Could you check a few things on this model? Use its own coordinates, in mm. A direction names the side the tool comes from. Round coordinates to 2 decimals unless told otherwise and drop trailing zeros. Loops run counter-clockwise (first coordinate to the right, second up) from the corner with the lowest first, then second, coordinate; pieces in that order, holes last.
from build123d import *

# Parameters (mm, degrees)
BOX_W           = 200
BOX_H           = 200
BOX_DEPTH       = 200
SKETCH_W        = 170.31563
SKETCH_H        = 140.120693
SKETCH_W_2      = 170.274007
SKETCH_H_2      = 27.404772
POCKET_DEPTH    = 180
SKETCH001_R     = 6
POCKET004_DEPTH = 20


with BuildPart() as part:
    # Box → Box (new body)
    with BuildSketch(Plane.XY):
        with Locations((100, 100)):
            Rectangle(BOX_W, BOX_H)
    extrude(amount=BOX_DEPTH)

    # Sketch → Pocket (cut)
    with BuildSketch(Plane.XZ):
        with Locations((99.987303, 117.884569)):
            Rectangle(SKETCH_W, SKETCH_H)
        with Locations((99.992803, 27.16207)):
            Rectangle(SKETCH_W_2, SKETCH_H_2)
    extrude(amount=-POCKET_DEPTH, mode=Mode.SUBTRACT)

    # Sketch001 → Pocket004 (cut)
    with BuildSketch(Plane.YZ.offset(200)):
        with Locations((130.008312, 66.836238)):
            Circle(SKETCH001_R)
        with Locations((160.008312, 66.836238)):
            Circle(SKETCH001_R)
    extrude(amount=-POCKET004_DEPTH, mode=Mode.SUBTRACT)


solid = part.part
Item 1: For faces 5 (the flat face through (99, 89, 187.945)), 6 (the flat face through (99, 101, 0)), 7 (the cylindrical face through (192.677, 155.247, 63.185)), which set-ups out of +Z, -Z, +X, -X, +Y, -Y let a thin tool reach every point of the face, with its end or its side?
Results list:
face 5: -Y
face 6: -Z, +X, -X, +Y, -Y
face 7: +X
Item 2: If we section it at A-A, the plane y = 133: Please give me the cut outline in (x, z).
Results list:
outline: (0, 0) - (200, 0) - (200, 61.64) - (185.15, 61.64) - (185.15, 47.82) - (14.83, 47.82) - (14.83, 187.94) - (185.15, 187.94) - (185.15, 72.04) - (200, 72.04) - (200, 200) - (0, 200) - close; hole (14.86, 13.46) - (185.13, 13.46) - (185.13, 40.86) - (14.86, 40.86) - close
Item 3: If I drill on line 1 along Z through (x, y) = (71, 68); line 2 along X through (y, z) = (81.5, 105); line 3 along X through (y, z) = (161, 17), over which ranges is the centre line in solid material (lowest first)?
Results list:
line 1: z = 0 to 13.46, 40.86 to 47.82, 187.94 to 200
line 2: x = 0 to 14.83, 185.15 to 200
line 3: x = 0 to 14.86, 185.13 to 200
Item 4: Will this pin go through, and if not, where does the flat tip stop? pin 1 (12 mm diameter, centred on x = 171.5, z = 149, fed in from -Y).
Results list:
pin 1: stops at y = 180
Item 5: If we section it at D-D, the plane z = 16.5: Please give me the cut outline in (x, y).
Results list:
outline: (0, 0) - (14.86, 0) - (14.86, 180) - (185.13, 180) - (185.13, 0) - (200, 0) - (200, 200) - (0, 200) - close
Item 6: If we section it at C-C, the plane z = 139: Please give me the cut outline in (x, y), then the cut area to 3 significant figures.
Results list:
outline: (0, 0) - (14.83, 0) - (14.83, 180) - (185.15, 180) - (185.15, 0) - (200, 0) - (200, 200) - (0, 200) - close
area: 9,340 mm2
Item 7: We'd pull the mould along Z, two halves only. Please class faces 1 (the flat face through (0, 99, 99)), 2 (the flat face through (99, 101, 200)), 3 (the cylindrical face through (192.677, 124.014, 67.1)), 4 (the flat face through (14.856, 89, 27)): released by +Z, released by -Z, zero draft, split by the parting line, or undercut.
Results list:
face 1: zero draft
face 2: released by +Z
face 3: undercut
face 4: undercut
Item 8: If we section it at B-B, the plane x = 21: Please give me the cut outline in (y, z).
Results list:
outline: (0, 0) - (200, 0) - (200, 200) - (0, 200) - (0, 187.94) - (180, 187.94) - (180, 47.82) - (0, 47.82) - (0, 40.86) - (180, 40.86) - (180, 13.46) - (0, 13.46) - close
